Could you check a few things on this model? Use its own coordinates, in mm. A direction names the side the tool comes from. Coordinates: 2 decimals unless noted, no trailing zeros. Loops run counter-clockwise (first coordinate to the right, second up) from the corner with the lowest first, then second, coordinate; pieces in that order, holes last.
from build123d import *

# Parameters (mm, degrees)
SALIENTE_EXTRUIR1_DEPTH = 15
CROQUIS2_R              = 2.5
CORTAR_EXTRUIR1_DEPTH   = 15


with BuildPart() as part:
    # Croquis1 → Saliente-Extruir1 (new body)
    with BuildSketch(Plane.XY):
        with BuildLine():
            Line((5.454356057, 2.5), (17.454356057, 2.5))
            ThreePointArc((17.454356057, 2.5), (44.62432265, 0), (17.454356057, -2.5))
            Line((17.454356057, -2.5), (13.54145622, -2.5))
            Line((13.54145622, -2.5), (9.54145622, -2.5))
            Line((9.54145622, -2.5), (5.454356057, -2.5))
            ThreePointArc((5.454356057, -2.5), (-6, 0), (5.454356057, 2.5))
        make_face()
        with BuildLine():
            Line((4.769696007, 1.5), (18.313216433, 1.5))
            ThreePointArc((18.313216433, 1.5), (43.62432265, 0), (18.313216433, -1.5))
            Line((18.313216433, -1.5), (13.54145622, -1.5))
            Line((13.54145622, -1.5), (9.54145622, -1.5))
            Line((9.54145622, -1.5), (4.769696007, -1.5))
            ThreePointArc((4.769696007, -1.5), (-5, 0), (4.769696007, 1.5))
        make_face(mode=Mode.SUBTRACT)
    extrude(amount=SALIENTE_EXTRUIR1_DEPTH)

    # Croquis2 → Cortar-Extruir1 (cut)
    with BuildSketch(Plane(origin=(0, 2.5, 0), x_dir=(1, 0, 0), z_dir=(0, 1, 0))):
        with Locations(Location((11.454356057, -7.5, 0), (0, 0, 270))):
            Circle(CROQUIS2_R)
    extrude(amount=-CORTAR_EXTRUIR1_DEPTH, mode=Mode.SUBTRACT)


solid = part.part
1) Imagine slicing it at B-B on z = 7.5. List the corners of the cut face in (x, y) for me, plus the area to 3 significant figures.
2) Will these pins go through, and if not, where does the flat tip stop? pin 1 (10 mm diameter, centred on x = 16, y = 0, fed in from +Z); pin 2 (4 mm diameter, centred on x = 12.5, z = 5, fed in from -Y); pin 3 (7 mm diameter, centred on x = 12, z = 5.5, fed in from +Y); pin 4 (8 mm diameter, centred on y = 7.5, z = 11.5, fed in from +X).
3) Imagine slicing it at C-C on x = 10. List the corners of the cut face in (y, z) for me, plus the area to 3 significant figures.
4) We'd pull the mould along Y, two halves only. Please class faces 1 (the cylindrical face through (-6, 0, 7)), 2 (the flat face through (15, -1.5, 7)), 3 (the flat face through (14.2, -2.5, 7.4)): released by +Y, released by -Y, zero draft, split by the parting line, or undercut.
5) If I drill on L1, parallel to Y at x = 8, z = 5.75; L2, parallel to X at y = 2.1, z = 7.5; L3, parallel to X at y = 2.35, z = 7.5 (3 decimals), over which ranges is the centre line in solid material (lowest first)?
6) Imagine slicing it at A-A on y = 0. List the corners of the cut face in (x, z) for me.
7) For faces 4 (the flat face through (8.7, 2.5, 7.4)), 5 (the flat face through (14.5, 1.5, 7.4)), 6 (the flat face through (18, -2, 15)), which set-ups out of +Z, -Z, +X, -X, +Y, -Y let a thin tool reach every point of the face, with its end or its side?
8) Imagine slicing it at D-D on x = 31. List the corners of the cut face in (y, z) for me, plus the area to 3 significant figures.
Solved:
1. outline: (4.77, -1.5) arc R5 cw (long way) to (4.77, 1.5) - (8.95, 1.5) - (8.95, 2.5) - (5.45, 2.5) arc R6 ccw (long way) to (5.45, -2.5) - (8.95, -2.5) - (8.95, -1.5) - close; (13.95, -2.5) - (17.45, -2.5) arc R13.7 ccw (long way) to (17.45, 2.5) - (13.95, 2.5) - (13.95, 1.5) - (18.31, 1.5) arc R12.7 cw (long way) to (18.31, -1.5) - (13.95, -1.5) - close
1. area: 125 mm2
2. pin 1: stops at z = 15
2. pin 2: stops at y = -2.5
2. pin 3: stops at y = 2.5
2. pin 4: stops at x = 44.17
3. outline: (-2.5, 0) - (-1.5, 0) - (-1.5, 5.47) - (-2.5, 5.47) - close; (-2.5, 9.53) - (-1.5, 9.53) - (-1.5, 15) - (-2.5, 15) - close; (1.5, 0) - (2.5, 0) - (2.5, 5.47) - (1.5, 5.47) - close; (1.5, 9.53) - (2.5, 9.53) - (2.5, 15) - (1.5, 15) - close
3. area: 21.9 mm2
4. face 1: split by the parting line
4. face 2: undercut
4. face 3: released by -Y
5. L1: y = -2.5 to -1.5, 1.5 to 2.5
5. L2: x = -5.62 to -4.54, 4.54 to 8.95, 13.95 to 18.4, 43.45 to 44.46
5. L3: x = -5.521 to -4.413, 4.413 to 8.954, 13.954 to 18.444, 43.405 to 44.421
6. outline: (-6, 0) - (-5, 0) - (-5, 15) - (-6, 15) - close; (43.62, 0) - (44.62, 0) - (44.62, 15) - (43.62, 15) - close
7. face 4: +Z, -Z, +Y
7. face 5: +Z, -Z
7. face 6: +Z, +X, -X, +Y, -Y
8. outline: (-13.7, 0) - (-12.7, 0) - (-12.7, 15) - (-13.7, 15) - close; (12.7, 0) - (13.7, 0) - (13.7, 15) - (12.7, 15) - close
8. area: 30.0 mm2
